Can you work these out from the model? Positions are in its coordinate system, mm. A direction names the side the tool comes from. Round coordinates to 2 decimals unless told otherwise and drop trailing zeros. Loops run counter-clockwise (first coordinate to the right, second up) from the corner with the lowest first, then second, coordinate; pieces in that order, holes last.
(1) Will these pins go through, and if not, where does the flat tip stop? pin 1 Ø2.5 at (x, z) = (13.78, 0.18) entering from +Y; pin 2 Ø1.5 at (y, z) = (24.5, -2.5) entering from -X; pin 3 Ø4 at (x, z) = (-14.5, 0) entering from -Y; pin 4 Ø2.5 at (y, z) = (23, -0.5) entering from +X.
(2) I want a section at C-C on y = 23.5. Write out the boundary of the cut face in (x, z).
(3) I want a section at B-B on z = 2.75. Write out the boundary of the cut face in (x, y).
(4) Which directions (+Z, -Z, +X, -X, +Y, -Y) give clear straight access to the entire face, cutting with the end or side of a thin tool? Please do faces 4 (the face through (-11.344, 11, 0)), 5 (the face through (-12.6, 21.435, -0.1)), 6 (the face through (12, 18.435, 0)), 7 (the face through (4.72, 32.41, -1.95)).
(5) Thinking about a two-plate mould opening in X: for faces 1 (the face through (-16.007, 19.914, -0.017)), 2 (the face through (-11.344, 24, 0)), 3 (the face through (3, 30.435, 0)), which applies, released by +X, released by -X, zero draft, split by the parting line, or undercut?
(6) I want a section at A-A on x = -8.5. Write out the boundary of the cut face in (y, z), plus the area to 3 significant figures.
(7) If I drill on line 1 along X through (y, z) = (18.5, 0); line 2 along Y through (x, z) = (11.5, -1.75); line 3 along X through (y, z) = (11, -3.75), over which ranges is the centre line in solid material (lowest first)?
Autodesk Inventor part; units mm, degrees
ref_plane "YZ Plane" through (0, 0, 0) normal (1, 0, 0) x (0, 1, 0)
ref_plane "XZ Plane" through (0, 0, 0) normal (0, 1, 0) x (-1, 0, 0)
ref_plane "XY Plane" through (0, 0, 0) normal (0, 0, 1) x (1, 0, 0)
sketch "Sketch1" plane through (0, 0, 0) normal (0, 0, 1) x (1, 0, 0)
  line L0 (-11.3443, 2.4351) -> (-0.3443, 2.4351)
  line L1 (-0.3443, 2.4351) -> (-0.3443, 26.4351)
  line L2 (-0.3443, 26.4351) -> (-11.3443, 26.4351)
  line L3 (-11.3443, 26.4351) -> (-11.3443, 2.4351)
  line L4 (-10.0022, 21.4351) -> (-10.0022, 22.9768)
  line L5 (-11.3443, 21.4351) -> (-16.0443, 21.4351)
  line L6 (-16.3443, 21.1351) -> (-16.3443, 18.7351)
  line L7 (-16.0443, 18.4351) -> (-11.3443, 18.4351)
  line L8 (10.6557, 2.4351) -> (-0.3443, 2.4351)
  line L9 (-0.3443, 26.4351) -> (10.6557, 26.4351)
  line L10 (10.6557, 26.4351) -> (10.6557, 2.4351)
  line L11 (10.6557, 21.4351) -> (15.3557, 21.4351)
  line L12 (15.6557, 21.1351) -> (15.6557, 18.7351)
  line L13 (15.3557, 18.4351) -> (10.6557, 18.4351)
  arc A0 (-16.3443, 18.7351) -> (-16.0443, 18.4351) centre (-16.0443, 18.7351) ccw
  arc A1 (-16.0443, 21.4351) -> (-16.3443, 21.1351) centre (-16.0443, 21.1351) ccw
  arc A2 (15.3557, 18.4351) -> (15.6557, 18.7351) centre (15.3557, 18.7351) ccw
  arc A3 (15.6557, 21.1351) -> (15.3557, 21.4351) centre (15.3557, 21.1351) ccw
  point P0 (0, 0)
  point P1 (-16.3443, 21.4351)
  point P2 (-16.3443, 18.4351)
  point P3 (15.6557, 21.4351)
  point P4 (15.6557, 18.4351)
  dimension "d0" = 11
  dimension "d1" = 24
  dimension "d3" = 5
  dimension "d4" = 3
  dimension "d5" = 0.3
extrude "Extrusion1" add sketch "Sketch1" along normal mid plane 11
sketch "Sketch2" plane through (-11.3443, 26.4351, 5.5) normal (0, 1, 0) x (1, 0, 0)
  line L0 (22, 11) -> (22, 0)
  arc A0 (11.1667, 4.1563) -> (11.1667, 6.8437) centre (16.5, 5.5) ccw
  arc A1 (11.1667, 6.8437) -> (11.1667, 4.1563) centre (10.5, 5.5) ccw
  point P0 (11.3443, 5.5)
  dimension "d9" = 11
  dimension "d11" = 3
extrude "Extrusion2" add sketch "Sketch2" along normal blind 4
sketch "Sketch3" plane through (-11.3443, 30.4351, 5.5) normal (0, 1, 0) x (1, 0, 0)
  line L0 (22, 11) -> (22, 5.5)
  circle A0 centre (16.5, 5.5) radius 2
  point P0 (11.3443, 5.5)
extrude "Extrusion3" add sketch "Sketch3" along normal blind 4
sketch "Sketch4" plane through (-16.0443, 21.4351, 5.5) normal (0, 1, 0) x (1, 0, 0)
  point P0 (16.0443, 5.5)
  point P1 (1.5246, 5.3219)
  point P2 (29.8245, 5.3219)
hole "Hole1" at (13.7802, 21.4351, 0.1781) at (-14.5197, 21.4351, 0.1781) direction (0, -1, 0) diameter 3 end through all
equation "\"BendRadius\" = Thickness"
equation "\"BendReliefWidth\" = Thickness"
equation "\"BendReliefDepth\" = 0.5 * Thickness"
equation "\"CornerReliefSize\" = 4 * Thickness"
equation "\"MinimumRemnant\" = 2 * Thickness"
equation "\"TransitionRadius\" = BendRadius"
equation "\"JacobiRadiusSize\" = Thickness"
equation "\"GapSize\" = Thickness"
properties part number "servo1" material "PBT Plastic"
Filled sheet:
1. pin 1: passes through
1. pin 2: stops at x = -11.34
1. pin 3: stops at y = 18.44
1. pin 4: stops at x = 10.66
2. outline: (-11.34, -5.5) - (10.66, -5.5) - (10.66, 5.5) - (-11.34, 5.5) - close
3. outline: (-16.34, 18.74) arc R0.3 ccw to (-16.04, 18.44) - (-11.34, 18.44) - (-11.34, 2.44) - (10.66, 2.44) - (10.66, 18.44) - (15.36, 18.44) arc R0.3 ccw to (15.66, 18.74) - (15.66, 21.14) arc R0.3 ccw to (15.36, 21.44) - (10.66, 21.44) - (10.66, 26.44) - (9.92, 26.44) - (9.92, 30.44) - (0.39, 30.44) - (0.39, 26.44) - (-11.34, 26.44) - (-11.34, 21.44) - (-16.04, 21.44) arc R0.3 ccw to (-16.34, 21.14) - close
4. face 4: +Z, -Z, -X, -Y
4. face 5: +Z, -Z, -X, +Y
4. face 6: +Z, -Z, +X, -Y
4. face 7: +Y
5. face 1: undercut
5. face 2: released by -X
5. face 3: zero draft
6. outline: (2.44, -5.5) - (26.44, -5.5) - (26.44, 5.5) - (2.44, 5.5) - close
6. area: 264 mm2
7. line 1: x = -16.23 to -16.01, -13.03 to 12.29, 15.27 to 15.54
7. line 2: y = 18.44 to 21.44
7. line 3: x = -11.34 to 10.66
